```python
from build123d import *

# Parameters (mm, degrees)
SKETCH1_W           = 32
SKETCH1_H           = 64
SKETCH1_R           = 4
SKETCH1_R_2         = 2
SKETCH1_R_3         = 1.6
BOSS_EXTRUDE1_DEPTH = 3
BOSS_EXTRUDE2_START = -3.05
SKETCH1_5_W         = 32
SKETCH1_5_H         = 64
SKETCH1_5_R         = 4
SKETCH1_5_R_2       = 2
BOSS_EXTRUDE2_DEPTH = 3.05
SKETCH2_W           = 64
SKETCH2_H           = 35.05
SKETCH2_R           = 4
SKETCH2_R_2         = 2
BOSS_EXTRUDE3_DEPTH = 3
CUT_EXTRUDE1_START  = -38.05
CUT_EXTRUDE1_DEPTH  = 35.05
CUT_EXTRUDE2_START  = -38.05
CUT_EXTRUDE2_DEPTH  = 35.05
RIB1_REACH          = 110.796
SKETCH4_WALL_W      = 269.16074152
SKETCH4_WALL_H      = 8


# Read off the part's stored shape, not the designer's step: Cut-Extrude1, Cut-Extrude2
with BuildPart() as part:
    # Sketch1 → Boss-Extrude1 (new body)
    # profile 1 of 2: a face of its own
    with BuildSketch(Plane(origin=(0, 0, 0), x_dir=(1, 0, 0), z_dir=(0, 1, 0))):
        with Locations((0, -16)):
            Rectangle(SKETCH1_W, SKETCH1_H)
        with Locations(Location((0, -32, 0), (0, 0, 270))):
            Circle(SKETCH1_R, mode=Mode.SUBTRACT)
        with Locations(Location((0, -40, 0), (0, 0, 270))):
            Circle(SKETCH1_R_2, mode=Mode.SUBTRACT)
        with Locations(Location((0, 0, 0), (0, 0, 270))):
            Circle(SKETCH1_R, mode=Mode.SUBTRACT)
        with Locations(Location((0, 8, 0), (0, 0, 270))):
            Circle(SKETCH1_R_2, mode=Mode.SUBTRACT)
        with Locations(Location((0, -16, 0), (0, 0, 270))):
            Circle(SKETCH1_R, mode=Mode.SUBTRACT)
        with Locations(Location((8, 0, 0), (0, 0, 270))):
            Circle(SKETCH1_R_2, mode=Mode.SUBTRACT)
        with Locations(Location((0, -8, 0), (0, 0, 270))):
            Circle(SKETCH1_R_2, mode=Mode.SUBTRACT)
        with Locations(Location((-8, 0, 0), (0, 0, 270))):
            Circle(SKETCH1_R_2, mode=Mode.SUBTRACT)
        with Locations(Location((-8, -32, 0), (0, 0, 270))):
            Circle(SKETCH1_R_2, mode=Mode.SUBTRACT)
        with Locations(Location((8, -32, 0), (0, 0, 270))):
            Circle(SKETCH1_R_2, mode=Mode.SUBTRACT)
        with Locations(Location((0, -24, 0), (0, 0, 270))):
            Circle(SKETCH1_R_2, mode=Mode.SUBTRACT)
    # profile 2 of 2: a face of its own
    with BuildSketch(Plane(origin=(0, 0, 0), x_dir=(1, 0, 0), z_dir=(0, 1, 0))):
        with BuildLine():
            ThreePointArc((16, 16), (31.762527334, 8.054271284), (48.722, 12.95))
            Line((48.722, 12.95), (48.722, 51.05))
            Line((48.722, 51.05), (78.182, 51.05))
            Line((78.182, 51.05), (78.182, 12.95))
            ThreePointArc((78.182, 12.95), (59.535915128, -30.221467801), (16, -48))
            Line((16, -48), (16, 16))
        make_face()
        with Locations(Location((71.452, 16, 0), (0, 0, 270))):
            Circle(SKETCH1_R_3, mode=Mode.SUBTRACT)
        with Locations(Location((71.452, 48, 0), (0, 0, 270))):
            Circle(SKETCH1_R_3, mode=Mode.SUBTRACT)
        with Locations(Location((55.452, 48, 0), (0, 0, 270))):
            Circle(SKETCH1_R_3, mode=Mode.SUBTRACT)
        with Locations(Location((55.452, 16, 0), (0, 0, 270))):
            Circle(SKETCH1_R_3, mode=Mode.SUBTRACT)
    extrude(amount=BOSS_EXTRUDE1_DEPTH)

    # Sketch1<5> → Boss-Extrude2 (add)
    with BuildSketch(Plane(origin=(0, 0, 0), x_dir=(1, 0, 0), z_dir=(0, 1, 0)).offset(BOSS_EXTRUDE2_START)):
        with Locations((0, -16)):
            Rectangle(SKETCH1_5_W, SKETCH1_5_H)
        with Locations(Location((0, -32, 0), (0, 0, 270))):
            Circle(SKETCH1_5_R, mode=Mode.SUBTRACT)
        with Locations(Location((0, -40, 0), (0, 0, 270))):
            Circle(SKETCH1_5_R_2, mode=Mode.SUBTRACT)
        with Locations(Location((0, 0, 0), (0, 0, 270))):
            Circle(SKETCH1_5_R, mode=Mode.SUBTRACT)
        with Locations(Location((0, 8, 0), (0, 0, 270))):
            Circle(SKETCH1_5_R_2, mode=Mode.SUBTRACT)
        with Locations(Location((0, -16, 0), (0, 0, 270))):
            Circle(SKETCH1_5_R, mode=Mode.SUBTRACT)
        with Locations(Location((8, 0, 0), (0, 0, 270))):
            Circle(SKETCH1_5_R_2, mode=Mode.SUBTRACT)
        with Locations(Location((0, -8, 0), (0, 0, 270))):
            Circle(SKETCH1_5_R_2, mode=Mode.SUBTRACT)
        with Locations(Location((-8, 0, 0), (0, 0, 270))):
            Circle(SKETCH1_5_R_2, mode=Mode.SUBTRACT)
        with Locations(Location((-8, -32, 0), (0, 0, 270))):
            Circle(SKETCH1_5_R_2, mode=Mode.SUBTRACT)
        with Locations(Location((8, -32, 0), (0, 0, 270))):
            Circle(SKETCH1_5_R_2, mode=Mode.SUBTRACT)
        with Locations(Location((0, -24, 0), (0, 0, 270))):
            Circle(SKETCH1_5_R_2, mode=Mode.SUBTRACT)
    extrude(amount=BOSS_EXTRUDE2_DEPTH)

    # Sketch2 → Boss-Extrude3 (add)
    with BuildSketch(Plane(origin=(16, 0, 0), x_dir=(0, 0, -1), z_dir=(1, 0, 0))):
        with Locations((-16, -17.525)):
            Rectangle(SKETCH2_W, SKETCH2_H)
        with Locations((0, -19.05)):
            Circle(SKETCH2_R, mode=Mode.SUBTRACT)
        with Locations((8, -19.05)):
            Circle(SKETCH2_R_2, mode=Mode.SUBTRACT)
        with Locations((0, -27.05)):
            Circle(SKETCH2_R_2, mode=Mode.SUBTRACT)
        with Locations((-8, -19.05)):
            Circle(SKETCH2_R_2, mode=Mode.SUBTRACT)
        with Locations((0, -11.05)):
            Circle(SKETCH2_R_2, mode=Mode.SUBTRACT)
        with Locations(Location((-32, -27.05, 0), (0, 0, 180))):
            Circle(SKETCH2_R_2, mode=Mode.SUBTRACT)
        with Locations(Location((-40, -19.05, 0), (0, 0, 180))):
            Circle(SKETCH2_R_2, mode=Mode.SUBTRACT)
        with Locations(Location((-24, -19.05, 0), (0, 0, 180))):
            Circle(SKETCH2_R_2, mode=Mode.SUBTRACT)
        with Locations(Location((-32, -11.05, 0), (0, 0, 180))):
            Circle(SKETCH2_R_2, mode=Mode.SUBTRACT)
        with Locations(Location((-32, -19.05, 0), (0, 0, 180))):
            Circle(SKETCH2_R, mode=Mode.SUBTRACT)
    extrude(amount=BOSS_EXTRUDE3_DEPTH)

    # Cut-Extrude1 outline → Cut-Extrude1 (cut)
    with BuildSketch(Plane(origin=(0, 3, 0), x_dir=(1, 0, 0), z_dir=(0, 1, 0)).offset(CUT_EXTRUDE1_START)):
        with BuildLine():
            ThreePointArc((16, 16), (17.439637495, 14.523053201), (19, 13.174277157))
            Line((19, 13.174277157), (19, 16))
            Line((19, 16), (16, 16))
        make_face()
    extrude(amount=CUT_EXTRUDE1_DEPTH, mode=Mode.SUBTRACT)

    # Cut-Extrude2 outline → Cut-Extrude2 (cut)
    with BuildSketch(Plane(origin=(0, 3, 0), x_dir=(1, 0, 0), z_dir=(0, 1, 0)).offset(CUT_EXTRUDE2_START)):
        with BuildLine():
            Line((16, -48), (19, -48))
            Line((19, -48), (19, -47.927604143))
            ThreePointArc((19, -47.927604143), (17.5004367, -47.981898402), (16, -48))
        make_face()
    extrude(amount=CUT_EXTRUDE2_DEPTH, mode=Mode.SUBTRACT)

    # Sketch4 wall → Rib1 (add, up to next)
    with BuildSketch(Plane(origin=(36.525, -17.525, 16), x_dir=(0.707106781187, 0.707106781187, 0), z_dir=(-0.707106781187, 0.707106781187, 0)), mode=Mode.PRIVATE) as rib1_sk1:
        Rectangle(SKETCH4_WALL_W, SKETCH4_WALL_H)
    rib1_tool1 = extrude(rib1_sk1.sketch, amount=RIB1_REACH, mode=Mode.PRIVATE) - part.part
    add(rib1_tool1.solids().sort_by_distance((36.525, -17.525, 16))[0])


solid = part.part
```
Verification items for the finished model (mm, model axes). A direction names the side the tool comes from. Coordinates: 2 decimals unless noted, no trailing zeros. Loops run counter-clockwise (first coordinate to the right, second up) from the corner with the lowest first, then second, coordinate; pieces in that order, holes last. Notation, with made-up numbers: (-23.5, 41) -> (-5.5, 41) arc R25 ccw to (-5.5, 71) -> close; hole circle Ø5 at (61.25, 40.5). An arc over 180 degrees is marked (long way). Answer in a Markdown table with one row per item.
1) Section check A-A (y = -11.05). Record the cut outline in (x, z), and give its area (3 significant figures).
The answers:
| item | result |
|---|---|
| outline | (16, -16) arc R24.16 cw to (19, -13.17) -> (19, -2) -> (16, -2) -> close; (16, 2) -> (19, 2) -> (19, 12) -> (43, 12) -> (43, 20) -> (19, 20) -> (19, 30) -> (16, 30) -> close; (16, 34) -> (19, 34) -> (19, 47.93) arc R62.19 ccw to (16, 48) -> close |
| area | 355 mm2 |
2) Scan lines: line 1 along Y through (x, z) = (18.35, 0); line 2 along Y through (x, z) = (18, -8); line 3 along X through (y, z) = (-31.5, 21). Record each from-to range of solid material in increasing order. Write a range as from..to.
The answers:
| item | result |
|---|---|
| line 1 | y = -35.05..-29.05, -25.05..-23.05, -15.05..-13.05, -9.05..3 |
| line 2 | y = -35.05..-21.05, -17.05..3 |
| line 3 | x = 16..19 |
3) Section check B-B (x = 8). Record the cut outline in (y, z), and give its area (3 significant figures).
The answers:
| item | result |
|---|---|
| outline | (-3.05, -16) -> (3, -16) -> (3, -2) -> (-3.05, -2) -> close; (-3.05, 2) -> (3, 2) -> (3, 30) -> (-3.05, 30) -> close; (-3.05, 34) -> (3, 34) -> (3, 48) -> (-3.05, 48) -> close |
| area | 339 mm2 |
4) Draft check along X on faces 4 (the face through (36.28, -17.77, 15.94)), 5 (the face through (8.601, -0.067, 33.908)), 6 (the face through (0, 0, 38)), 7 (the face through (49, 0, -2)). Enter one of: released by +X, released by -X, zero draft, split by the parting line, or undercut.
The answers:
| item | result |
|---|---|
| face 4 | released by +X |
| face 5 | undercut |
| face 6 | undercut |
| face 7 | zero draft |
5) Access from +Z, -Z, +X, -X, +Y, -Y to the whole of each face (thin tool, end or side, straight path). Record for faces 1 (the face through (-7, -3.05, 16)), 2 (the face through (17.479, -15.084, 0.521)), 3 (the face through (30, -11, 12)).
The answers:
| item | result |
|---|---|
| face 1 | +Z, -Z, -X, -Y |
| face 2 | +X, -X |
| face 3 | -Z, +X, -Y |
6) Depth check by flat-ended pin: P1, Ø3, axis at y = -24.5, z = 19, coming from the -X side; P2, Ø1.5, axis at y = 1, z = -35, coming from the -X side; P3, Ø13, axis at x = 0, z = 0, coming from the -Y side; P4, Ø2.5, axis at x = 55.452, z = -48, coming from the +Y side. Enter the tip coordinate at first touch or a pass-through.
The answers:
| item | result |
|---|---|
| P1 | stops at x = 16 |
| P2 | stops at x = 48.72 |
| P3 | stops at y = -3.05 |
| P4 | passes through |
7) Section check D-D (z = 16). Record the cut outline in (x, y).
The answers:
| item | result |
|---|---|
| outline | (-16, -3.05) -> (-4, -3.05) -> (-4, 3) -> (-16, 3) -> close; (4, -3.05) -> (16, -3.05) -> (16, -35.05) -> (19, -35.05) -> (54.05, 0) -> (70.37, 0) -> (70.37, 3) -> (4, 3) -> close |
8) Section check C-C (y = -19.05). Give the number of separate pieces and of enclosed holes in the cut face, and give its area (3 significant figures).
The answers:
| item | result |
|---|---|
| separate pieces | 7 |
| enclosed holes | 0 |
| area | 219 mm2 |
